from build123d import *

# Parameters (mm, degrees)
SZKIC1_R                               = 15
DODANIE_WYCI_GNI_CIE1_DEPTH            = 36
SZKIC3_R                               = 21
SZKIC3_R_2                             = 11.115
DODANIE_WYCI_GNI_CIE2_DEPTH            = 20
DODANIE_WYCI_GNI_CIE4_START            = -17
SZKIC5_R                               = 11.115
DODANIE_WYCI_GNI_CIE4_DEPTH            = 17
ZAOKR_GLENIE1_R                        = 10
DODANIE_WYCI_GNI_CIE3_DEPTH            = 72
ZAOKR_GLENIE2_R                        = 8
WYTNIJ_WYCI_GNI_CIE1_REACH             = 136.093
SZKIC6_R                               = 10
WYTNIJ_WYCI_GNI_CIE1_DIRECTION_2_DEPTH = 135.093251135


with BuildPart() as part:
    # Szkic1 → Dodanie-wyciągnięcie1 (new body)
    with BuildSketch(Plane.XY):
        Circle(SZKIC1_R)
        with BuildLine():
            Line((-2.39, 10.855004606), (-2.39, 12.465))
            Line((-2.39, 12.465), (2.39, 12.465))
            Line((2.39, 12.465), (2.39, 10.855004606))
            ThreePointArc((2.39, 10.855004606), (8.663373333, 6.963417803), (11.115, 0))
            ThreePointArc((11.115, 0), (-6.963417803, -8.663373333), (-2.39, 10.855004606))
        make_face(mode=Mode.SUBTRACT)
    extrude(amount=DODANIE_WYCI_GNI_CIE1_DEPTH)

    # Szkic3 → Dodanie-wyciągnięcie2 (add)
    with BuildSketch(Plane.XY.offset(36)):
        Circle(SZKIC3_R)
        with Locations(Location((0, 0, 0), (0, 0, 102.416978829))):
            Circle(SZKIC3_R_2, mode=Mode.SUBTRACT)
    extrude(amount=DODANIE_WYCI_GNI_CIE2_DEPTH)

    # Szkic5 → Dodanie-wyciągnięcie4 (add)
    with BuildSketch(Plane.XY.offset(56).offset(DODANIE_WYCI_GNI_CIE4_START)):
        with Locations(Location((0, 0, 0), (0, 0, 102.416978829))):
            Circle(SZKIC5_R)
    extrude(amount=DODANIE_WYCI_GNI_CIE4_DEPTH)

    # Zaokrąglenie1
    # the kernel refuses this fillet: 10 mm, written as the material it adds along each edge
    with BuildSketch(Plane(origin=(0, 0, 36), x_dir=(1, 0, 0), z_dir=(0, -1, 0))) as zaokr_glenie1_piece_1:
        with BuildLine():
            CenterArc((25, -9.16515139), ZAOKR_GLENIE1_R, 113.578178478, 66.421821522)
            Line((21, 0), (20.92, 0.183303028))
            ThreePointArc((20.92, 0.183303028), (18, 0.2), (15, 0.2))
            Line((15, 0.2), (14.8, 0))
            Line((14.8, 0), (14.8, -9.16515139))
            Line((14.8, -9.16515139), (15, -9.16515139))
        make_face()
    revolve(axis=Axis((0, 0, 36), (0, 0, 1)))

    # Szkic4 → Dodanie-wyciągnięcie3 (add)
    with BuildSketch(Plane.XY.offset(56)):
        with BuildLine():
            Line((-12.492422502, 16.880147512), (-12.492422502, 13))
            Line((-12.492422502, 13), (12.492422502, 13))
            Line((12.492422502, 13), (12.492422502, 16.880147512))
            ThreePointArc((12.492422502, 16.880147512), (0, 21), (-12.492422502, 16.880147512))
        make_face()
        with BuildLine():
            Line((12.492422502, -13), (-12.492422502, -13))
            Line((-12.492422502, -13), (-12.492422502, -16.880147512))
            ThreePointArc((-12.492422502, -16.880147512), (0, -21), (12.492422502, -16.880147512))
            Line((12.492422502, -16.880147512), (12.492422502, -13))
        make_face()
    extrude(amount=DODANIE_WYCI_GNI_CIE3_DEPTH)

    # Zaokrąglenie2
    zaokr_glenie2_edges = [part.edges().sort_by_distance(p)[0] for p in [
        (0, 13, 56),
        (0, -13, 56),
    ]]
    fillet(zaokr_glenie2_edges, radius=ZAOKR_GLENIE2_R)

    # Szkic6 → Wytnij-wyciągnięcie1 (cut, up to next)
    with BuildSketch(Plane(origin=(0, -13, 0), x_dir=(1, 0, 0), z_dir=(0, 1, 0)), mode=Mode.PRIVATE) as wytnij_wyci_gni_cie1_sk1:
        with Locations(Location((0, -113, 0), (0, 0, 270))):
            Circle(SZKIC6_R)
    wytnij_wyci_gni_cie1_tool1 = extrude(wytnij_wyci_gni_cie1_sk1.sketch, amount=-WYTNIJ_WYCI_GNI_CIE1_REACH, mode=Mode.PRIVATE) & part.part
    add(wytnij_wyci_gni_cie1_tool1.solids().sort_by_distance((0, -13, 113))[0], mode=Mode.SUBTRACT)

    # Szkic6 → Wytnij-wyciągnięcie1 direction 2 (cut)
    with BuildSketch(Plane(origin=(0, -13, 0), x_dir=(1, 0, 0), z_dir=(0, 1, 0))):
        with Locations(Location((0, -113, 0), (0, 0, 270))):
            Circle(SZKIC6_R)
    extrude(amount=WYTNIJ_WYCI_GNI_CIE1_DIRECTION_2_DEPTH, mode=Mode.SUBTRACT)


solid = part.part
Model file for the job. Use its own axes, mm. A direction names the side the tool comes from. Coordinates: 2 decimals unless noted, no trailing zeros. Write each loop counter-clockwise with the first axis right and the second up, starting at its lowest first coordinate (ties: lowest second). Pieces come first, ordered by that corner, then holes. Notation, with made-up numbers: (24.25, -2.5) -> (49.25, -2.5) arc R19 ccw to (49.25, 8.5) -> close; hole circle Ø10 at (82.5, 80.25). An arc over 180 degrees is marked (long way). One line per item, written item: value. Start each with the question number.
1) Slice it at A-A on x = 0. Write the cut outline in (y, z) (3 decimals), then the cut area to 3 significant figures.
2) Probe probe 1 along Y at (x, z) = (0, 36.95) (3 decimals); probe 2 along Z at (x, y) = (0, -14.5). List the from-to ranges inside material, lowest first.
3) Which spindle directions (+Z, -Z, +X, -X, +Y, -Y) get a long thin tool onto all of the face, cutting with end or side? Do faces 1 (the face through (12.492, -14, 92)), 2 (the face through (-14.985, 0.66, 13.23)), 3 (the face through (-12.492, 14, 92)), 4 (the face through (0, 16, 128)), 5 (the face through (0, 13, 88)). Say none if no direction does.
4) Flat gauge pins, fed straight in: pin 1 Ø3.5 at (y, z) = (-13, 81.5) entering from +X; pin 2 Ø3.5 at (y, z) = (11.5, 104.5) entering from -X; pin 3 Ø4 at (x, y) = (-6, 3) entering from -Z. Where does each tip first touch, or does it go through?
5) Pull direction Z, two halves, no side cores. Call faces 6 (the face through (0, -13, 88)), 7 (the face through (-3.83, -16.055, 122.237)), 8 (the face through (0, 0, 56)), 9 (the face through (3, -11, 0)): +Z half, -Z half, draft (parallel to the pull), parting line (faces both ways), or undercut.
6) Slice it at B-B on z = 113. Write the cut outline in (x, y), then the cut area to 3 significant figures.
Answers follow:
1. outline: (-21, 36) arc R10 cw to (-15, 26.835) -> (-15, 0) -> (-11.115, 0) -> (-11.115, 39) -> (11.115, 39) -> (11.115, 36) -> (12.465, 36) -> (12.465, 0) -> (15, 0) -> (15, 26.835) arc R10 cw to (21, 36) -> (21, 103) -> (13, 103) -> (13, 64) arc R8 cw to (5, 56) -> (-5, 56) arc R8 cw to (-13, 64) -> (-13, 103) -> (-21, 103) -> close; (-21, 123) -> (-13, 123) -> (-13, 128) -> (-21, 128) -> close; (13, 123) -> (21, 123) -> (21, 128) -> (13, 128) -> close
1. area: 1,890 mm2
2. probe 1: -21 to -11.115, 11.115 to 21
2. probe 2: 0 to 103, 123 to 128
3. face 1: +Z, +X, +Y, -Y
3. face 2: -Z
3. face 3: +Z, -X, +Y, -Y
3. face 4: +Z, +X, -X, +Y, -Y
3. face 5: +Z, +X, -X
4. pin 1: x = 12.49
4. pin 2: x = -12.49
4. pin 3: z = 39
5. face 6: draft
5. face 7: undercut
5. face 8: +Z half
5. face 9: -Z half
6. outline: (-12.49, -16.88) arc R21 ccw to (-10, -18.47) -> (-10, -13) -> (-12.49, -13) -> close; (-12.49, 13) -> (-10, 13) -> (-10, 18.47) arc R21 ccw to (-12.49, 16.88) -> close; (10, -18.47) arc R21 ccw to (12.49, -16.88) -> (12.49, -13) -> (10, -13) -> close; (10, 13) -> (12.49, 13) -> (12.49, 16.88) arc R21 ccw to (10, 18.47) -> close
6. area: 47.0 mm2
